The figure shows three views and two pictorial views of one solid part (mm, origin at its lowest corner). Answer the questions. Coordinates: 2 decimals unless noted, no trailing zeros. Order: outer loops, then holes, each group sorted by start corner. A loop starts at its lowest first (then second) coordinate and runs counter-clockwise, first axis right, second up.
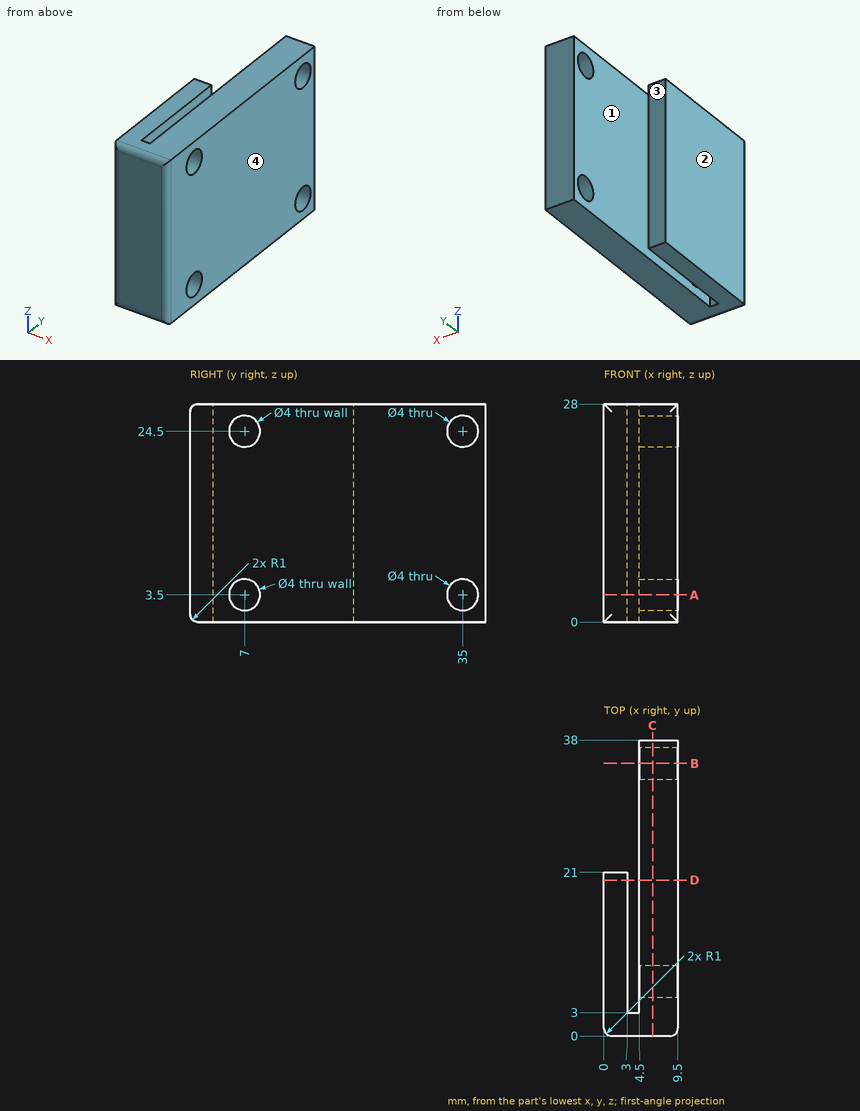
Q1. Each of these flat-tipped pins is pushed along its axis until it touches: P1, Ø3, axis at y = 35, z = 3.5, coming from the +X side; P2, Ø3.5, axis at x = 1.5, z = 12.5, coming from the +Y side. Where does it stop, or does it pass through?
Q2. Determine the mould class of the marked faces 1, 2, 3 and 4 for opening direction X: +X half, -X half, draft (parallel to the pull), parting line (faces both ways), or undercut.
Q3. The part is cut by section A-A, the plane z = 3.5. Determine the outline of the cut face in (x, y).
Q4. The part is cut by section D-D, the plane y = 20. Determine the outline of the cut face in (x, z), then the cut area to 3 significant figures.
Q5. The part is cut by section C-C, the plane x = 6.25. Determine the outline of the cut face in (y, z), then the cut area to 3 significant figures.
Q6. Straight lines are drawn through the part: L1, parallel to Z at x = 6.9, y = 7; L2, parallel to X at y = 19, z = 2.5; L3, parallel to Y at x = 2.25, z = 5.75. For each, find the intervals that lie inside material, in ascending order.
Q7. The part is cut by section B-B, the plane y = 35. Determine the outline of the cut face in (x, z), then the cut area to 3 significant figures.
Computed values:
1. P1: passes through
1. P2: stops at y = 21
2. face 1: undercut
2. face 2: -X half
2. face 3: draft
2. face 4: +X half
3. outline: (0, 1) arc R1 ccw to (1, 0) - (8.5, 0) arc R1 ccw to (9.5, 1) - (9.5, 5) - (4.5, 5) - (4.5, 3) - (3, 3) - (3, 21) - (0, 21) - close; (4.5, 9) - (9.5, 9) - (9.5, 33) - (4.5, 33) - close; (4.5, 37) - (9.5, 37) - (9.5, 38) - (4.5, 38) - close
4. outline: (0, 0) - (3, 0) - (3, 28) - (0, 28) - close; (4.5, 0) - (9.5, 0) - (9.5, 28) - (4.5, 28) - close
4. area: 224 mm2
5. outline: (0, 1) arc R1 ccw to (1, 0) - (38, 0) - (38, 28) - (1, 28) arc R1 ccw to (0, 27) - close; hole circle Ø4 at (7, 3.5); hole circle Ø4 at (7, 24.5); hole circle Ø4 at (35, 3.5); hole circle Ø4 at (35, 24.5)
5. area: 1,010 mm2
6. L1: z = 0 to 1.5, 5.5 to 22.5, 26.5 to 28
6. L2: x = 0 to 3, 4.5 to 9.5
6. L3: y = 0 to 21
7. outline: (4.5, 0) - (9.5, 0) - (9.5, 1.5) - (4.5, 1.5) - close; (4.5, 5.5) - (9.5, 5.5) - (9.5, 22.5) - (4.5, 22.5) - close; (4.5, 26.5) - (9.5, 26.5) - (9.5, 28) - (4.5, 28) - close
7. area: 100 mm2
